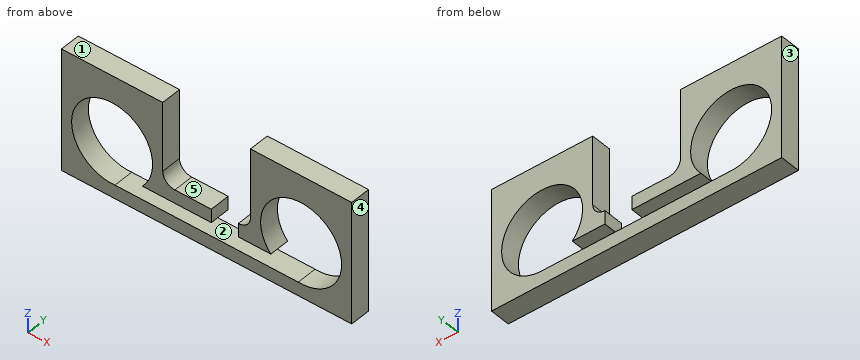
```python
from build123d import *

# Parameters (mm, degrees)
F0_W     = 273.05
F0_H     = 114.3
F1_DEPTH = 19.05
F2_R     = 38.1
F3_DEPTH = 25.4
F5_DEPTH = 25.4
F7_DEPTH = 25.4


with BuildPart() as f1:
    # F0 (on Front) → F1 (new body)
    with BuildSketch(Plane.XZ):
        with Locations((136.525, 57.15)):
            Rectangle(F0_W, F0_H)
    extrude(amount=F1_DEPTH)

    # F2 (on face) → F3 (cut)
    with BuildSketch(Plane.XZ.offset(19.05)):
        with Locations((225.425, 50.8)):
            Circle(F2_R)
        with Locations((47.625, 50.8)):
            Circle(F2_R)
    extrude(amount=-F3_DEPTH, mode=Mode.SUBTRACT)

    # F4 (on face) → F5 (cut)
    with BuildSketch(Plane.XZ.offset(19.05)):
        with BuildLine():
            Line((177.8, 114.3), (95.25, 114.3))
            Line((95.25, 114.3), (95.25, 49.53))
            ThreePointArc((95.25, 49.53), (98.597769, 41.447769), (106.68, 38.1))
            Line((106.68, 38.1), (166.37, 38.1))
            ThreePointArc((166.37, 38.1), (174.452231, 41.447769), (177.8, 49.53))
            Line((177.8, 49.53), (177.8, 114.3))
        make_face()
    extrude(amount=-F5_DEPTH, mode=Mode.SUBTRACT)

    # F6 (on face) → F7 (cut)
    with BuildSketch(Plane.XZ.offset(19.05)):
        Polygon((166.37, 25.494051), (166.37, 38.1), (140.97, 38.1), (140.97, 25.494051), (76.106905, 25.494051), (50.300408, 12.794051), (228.100408, 12.794051), (196.943095, 25.494051), align=None)
    extrude(amount=-F7_DEPTH, mode=Mode.SUBTRACT)


solid = f1.part
```
Work out the finished part from the listing and answer in its coordinate system (mm). Face numbers are marked on the shaded views. A direction names the side the tool comes from. Give positions to 0.01 mm unless a question says otherwise; leave off trailing zeros. Order: outer loops, then holes, each group sorted by start corner. A loop starts at its lowest first (then second) coordinate and runs counter-clockwise, first axis right, second up.
1. For the marked faces 4 and 5, determine the directions among +Z, -Z, +X, -X, +Y, -Y from which every point of the face is accessible in a straight line to the end or side of a thin tool.
Result sheet:
face 4: +Z, -Z, +X, +Y, -Y
face 5: +Z, +Y, -Y
2. This flat-tipped pin is pushed along its axis until it touches: P1, Ø9.5, axis at x = 122.5, y = -12, coming from the +Z side. Where does it stop, or does it pass through?
Result sheet:
P1: stops at z = 38.1
3. Section D-D, the plane z = 55.5 is taken. Determine the outline of the cut face in (x, y).
Result sheet:
outline: (0, -19.05) - (9.82, -19.05) - (9.82, 0) - (0, 0) - close; (85.43, -19.05) - (95.25, -19.05) - (95.25, 0) - (85.43, 0) - close; (177.8, -19.05) - (187.62, -19.05) - (187.62, 0) - (177.8, 0) - close; (263.23, -19.05) - (273.05, -19.05) - (273.05, 0) - (263.23, 0) - close
4. The mould has two halves that part along X. Classify the marked faces 1, 2 and 3: released by +X, released by -X, zero draft, split by the parting line, or undercut.
Result sheet:
face 1: zero draft
face 2: undercut
face 3: released by -X
5. Section C-C, the plane x = 252.5 is taken. Determine the outline of the cut face in (y, z).
Result sheet:
outline: (-19.05, 0) - (0, 0) - (0, 23.99) - (-19.05, 23.99) - close; (-19.05, 77.61) - (0, 77.61) - (0, 114.3) - (-19.05, 114.3) - close
6. Section A-A, the plane z = 97 is taken. Determine the outline of the cut face in (x, y).
Result sheet:
outline: (0, -19.05) - (95.25, -19.05) - (95.25, 0) - (0, 0) - close; (177.8, -19.05) - (273.05, -19.05) - (273.05, 0) - (177.8, 0) - close
7. Section B-B, the plane y = -11.75 is taken. Determine the outline of the cut face in (x, z) (3 decimals).
Result sheet:
outline: (0, 0) - (273.05, 0) - (273.05, 114.3) - (177.8, 114.3) - (177.8, 49.53) arc R11.43 cw to (166.37, 38.1) - (166.37, 25.494) - (196.943, 25.494) arc R38.1 cw (long way) to (222.75, 12.794) - (50.3, 12.794) arc R38.1 cw (long way) to (76.107, 25.494) - (140.97, 25.494) - (140.97, 38.1) - (106.68, 38.1) arc R11.43 cw to (95.25, 49.53) - (95.25, 114.3) - (0, 114.3) - close
8. Straight lines are drawn through the part: L1, parallel to X at y = -4.5, z = 50.8 (3 decimals); L2, parallel to Z at x = 127, y = -8.75; L3, parallel to Z at x = 179.5, y = -9.5. For each, find the intervals that lie inside material, in ascending order.
Result sheet:
L1: x = 0 to 9.525, 85.725 to 95.25, 177.8 to 187.325, 263.525 to 273.05
L2: z = 0 to 12.79, 25.49 to 38.1
L3: z = 0 to 12.79, 25.49 to 114.3
